Part model, mm, in its own coordinate system. Face numbers are marked on the shaded views. Coordinates: 2 decimals unless noted, no trailing zeros. Write each loop counter-clockwise with the first axis right and the second up, starting at its lowest first coordinate (ties: lowest second). Pieces come first, ordered by that corner, then holes. Notation, with made-up numbers: (-1, 30.5) -> (15, 30.5) arc R11 ccw to (15, 40.5) -> close; hole circle Ø5 at (28.5, -11). An arc over 180 degrees is marked (long way). Write item = value, one per line.
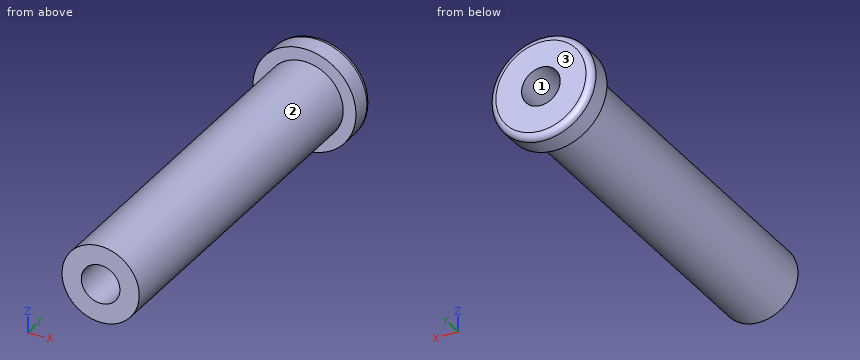
from build123d import *

# Parameters (mm, degrees)
SCHIZZO1_R                   = 6
SCHIZZO1_R_2                 = 3
ESTRUSIONE_ESTRUSIONE1_DEPTH = 56
SCHIZZO2_R                   = 8
SCHIZZO2_R_2                 = 3
ESTRUSIONE_ESTRUSIONE2_DEPTH = 4
RACCORDO1_R                  = 1


with BuildPart() as part:
    # Schizzo1 → Estrusione-Estrusione1 (new body)
    with BuildSketch(Plane(origin=(0, 0, 0), x_dir=(1, 0, 0), z_dir=(0, 1, 0))):
        Circle(SCHIZZO1_R)
        Circle(SCHIZZO1_R_2, mode=Mode.SUBTRACT)
    extrude(amount=ESTRUSIONE_ESTRUSIONE1_DEPTH)

    # Schizzo2 → Estrusione-Estrusione2 (add)
    with BuildSketch(Plane(origin=(0, 56, 0), x_dir=(1, 0, 0), z_dir=(0, 1, 0))):
        Circle(SCHIZZO2_R)
        Circle(SCHIZZO2_R_2, mode=Mode.SUBTRACT)
    extrude(amount=ESTRUSIONE_ESTRUSIONE2_DEPTH)

    # Raccordo1
    raccordo1_edges = [part.edges().sort_by_distance(p)[0] for p in [
        (-8, 60, 0),
    ]]
    fillet(raccordo1_edges, radius=RACCORDO1_R)


solid = part.part
Q1. Pin check, flat tips, straight feed: pin 1 (5 mm diameter, centred on x = 3.5, z = -1.5, fed in from -Y); pin 2 (3 mm diameter, centred on y = 11.5, z = 6, fed in from -X); pin 3 (5 mm diameter, centred on x = -2, y = 14, fed in from -Z); pin 4 (5 mm diameter, centred on x = 0, z = 0, fed in from -Y). Stop position of each tip, or through.
Model answer:
pin_1 = 0
pin_2 = -3.97
pin_3 = -6
pin_4 = through
Q2. Saw through at C-C on y = 18. Give the cut face in (x, z).
Model answer:
outline = circle Ø12 at (0, 0); hole circle Ø6 at (0, 0)
Q3. Saw through at A-A on x = 0. Give the cut face in (y, z).
Model answer:
outline = (0, -6) -> (56, -6) -> (56, -8) -> (59, -8) arc R1 ccw to (60, -7) -> (60, -3) -> (0, -3) -> close; (0, 3) -> (60, 3) -> (60, 7) arc R1 ccw to (59, 8) -> (56, 8) -> (56, 6) -> (0, 6) -> close
Q4. Probe line 1 (X direction, y = 24, z = 0); line 2 (Z direction, x = -2.75, y = 55). List the from-to ranges inside material, lowest first. Write a range as from..to.
Model answer:
line_1 = -6..-3, 3..6
line_2 = -5.33..-1.2, 1.2..5.33
Q5. Saw through at B-B on z = 0. Give the cut face in (x, y).
Model answer:
outline = (-8, 56) -> (-6, 56) -> (-6, 0) -> (-3, 0) -> (-3, 60) -> (-7, 60) arc R1 ccw to (-8, 59) -> close; (3, 0) -> (6, 0) -> (6, 56) -> (8, 56) -> (8, 59) arc R1 ccw to (7, 60) -> (3, 60) -> close
Q6. Mould opens along Z. For the marked faces 1, 2 and 3 say: released by +Z, released by -Z, zero draft, split by the parting line, or undercut.
Model answer:
face_1 = undercut
face_2 = split by the parting line
face_3 = zero draft
